Read the model definition and answer for the solid it produces. Units are mm, in the model's axes. Face numbers are marked on the shaded views. Round coordinates to 2 decimals unless told otherwise and drop trailing zeros. Loops run counter-clockwise (first coordinate to the right, second up) from the corner with the lowest first, then second, coordinate; pieces in that order, holes last. Notation, with made-up numbers: M -22,-33 L -9,-33 A23 ccw -9,1 Z; hole C 7,-14.75 d1. An arc over 180 degrees is marked long. Write each question's results on one line, items separated by ' | '.
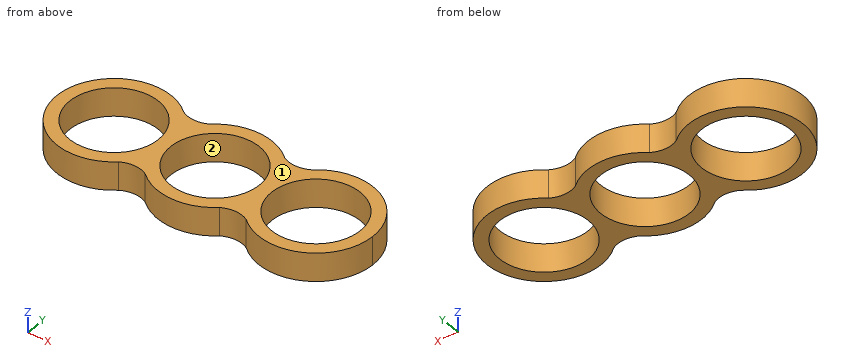
```python
from build123d import *

# Parameters (mm, degrees)
F0_R     = 11
F1_DEPTH = 7


with BuildPart() as f1:
    # F0 (on Top) → F1 (new body)
    with BuildSketch(Plane.XY):
        with BuildLine():
            ThreePointArc((-12.7, -6.29608), (-13.801325, -3.233274), (-14.175, 0))
            ThreePointArc((-14.175, 0), (-13.801325, 3.233274), (-12.7, 6.29608))
            ThreePointArc((-12.7, 6.29608), (-14.150621, 8.624506), (-16.022588, 10.6299))
            ThreePointArc((-16.022588, 10.6299), (-39.574997, 0.009606), (-16.037004, -10.6426))
            ThreePointArc((-16.037004, -10.6426), (-14.156468, -8.632127), (-12.7, -6.29608))
        make_face()
        with Locations((-25.4, 0)):
            Circle(F0_R, mode=Mode.SUBTRACT)
        with BuildLine():
            Line((11.225, 0), (11, 0))
            ThreePointArc((11, 0), (0, -11), (-11, 0))
            Line((-11, 0), (-11.225, 0))
            ThreePointArc((-11.225, 0), (-11.598675, -3.233274), (-12.7, -6.29608))
            ThreePointArc((-12.7, -6.29608), (-11.243532, -8.632127), (-9.362996, -10.6426))
            ThreePointArc((-9.362996, -10.6426), (0, -14.175), (9.362996, -10.6426))
            ThreePointArc((9.362996, -10.6426), (11.243532, -8.632127), (12.7, -6.29608))
            ThreePointArc((12.7, -6.29608), (11.598675, -3.233274), (11.225, 0))
        make_face()
        with BuildLine():
            ThreePointArc((-16.022588, 10.6299), (-14.150621, 8.624506), (-12.7, 6.29608))
            ThreePointArc((-12.7, 6.29608), (-11.243532, 8.632127), (-9.362996, 10.6426))
            ThreePointArc((-9.362996, 10.6426), (-12.691091, 9.744086), (-16.022588, 10.6299))
        make_face()
        with BuildLine():
            ThreePointArc((-12.7, -6.29608), (-11.598675, -3.233274), (-11.225, 0))
            Line((-11.225, 0), (-14.175, 0))
            ThreePointArc((-14.175, 0), (-13.801325, -3.233274), (-12.7, -6.29608))
        make_face()
        with BuildLine():
            Line((-14.175, 0), (-11.225, 0))
            ThreePointArc((-11.225, 0), (-11.598675, 3.233274), (-12.7, 6.29608))
            ThreePointArc((-12.7, 6.29608), (-13.801325, 3.233274), (-14.175, 0))
        make_face()
        with BuildLine():
            ThreePointArc((-11, 0), (0, 11), (11, 0))
            Line((11, 0), (11.225, 0))
            ThreePointArc((11.225, 0), (11.598675, 3.233274), (12.7, 6.29608))
            ThreePointArc((12.7, 6.29608), (11.243532, 8.632127), (9.362996, 10.6426))
            ThreePointArc((9.362996, 10.6426), (0, 14.175), (-9.362996, 10.6426))
            ThreePointArc((-9.362996, 10.6426), (-11.243532, 8.632127), (-12.7, 6.29608))
            ThreePointArc((-12.7, 6.29608), (-11.598675, 3.233274), (-11.225, 0))
            Line((-11.225, 0), (-11, 0))
        make_face()
        with BuildLine():
            ThreePointArc((-9.362996, -10.6426), (-11.243532, -8.632127), (-12.7, -6.29608))
            ThreePointArc((-12.7, -6.29608), (-14.156468, -8.632127), (-16.037004, -10.6426))
            ThreePointArc((-16.037004, -10.6426), (-12.7, -9.7536), (-9.362996, -10.6426))
        make_face()
        with BuildLine():
            ThreePointArc((16.037004, -10.6426), (14.156468, -8.632127), (12.7, -6.29608))
            ThreePointArc((12.7, -6.29608), (11.243532, -8.632127), (9.362996, -10.6426))
            ThreePointArc((9.362996, -10.6426), (12.7, -9.7536), (16.037004, -10.6426))
        make_face()
        with BuildLine():
            ThreePointArc((12.7, 6.29608), (13.801325, 3.233274), (14.175, 0))
            ThreePointArc((14.175, 0), (13.801325, -3.233274), (12.7, -6.29608))
            ThreePointArc((12.7, -6.29608), (14.156468, -8.632127), (16.037004, -10.6426))
            ThreePointArc((16.037004, -10.6426), (31.239955, -12.916096), (39.575, 0))
            ThreePointArc((39.575, 0), (31.239955, 12.916096), (16.037004, 10.6426))
            ThreePointArc((16.037004, 10.6426), (14.156468, 8.632127), (12.7, 6.29608))
        make_face()
        with BuildLine():
            ThreePointArc((36.4, 0), (25.4, -11), (14.4, 0))
            ThreePointArc((14.4, 0), (25.4, 11), (36.4, 0))
        make_face(mode=Mode.SUBTRACT)
        with BuildLine():
            ThreePointArc((12.7, 6.29608), (11.598675, 3.233274), (11.225, 0))
            Line((11.225, 0), (14.175, 0))
            ThreePointArc((14.175, 0), (13.801325, 3.233274), (12.7, 6.29608))
        make_face()
        with BuildLine():
            Line((14.175, 0), (11.225, 0))
            ThreePointArc((11.225, 0), (11.598675, -3.233274), (12.7, -6.29608))
            ThreePointArc((12.7, -6.29608), (13.801325, -3.233274), (14.175, 0))
        make_face()
        with BuildLine():
            ThreePointArc((9.362996, 10.6426), (11.243532, 8.632127), (12.7, 6.29608))
            ThreePointArc((12.7, 6.29608), (14.156468, 8.632127), (16.037004, 10.6426))
            ThreePointArc((16.037004, 10.6426), (12.7, 9.7536), (9.362996, 10.6426))
        make_face()
    extrude(amount=F1_DEPTH)


solid = f1.part
```
1. Find section C-C, the plane z = 2.75. Give the vertices of the cut face in (x, y) (3 decimals).
Completed:
outline: M -16.037,-10.643 A6.707 cw -9.363,-10.643 A14.175 ccw 9.363,-10.643 A6.707 cw 16.037,-10.643 A14.175 ccw 39.575,0 A14.175 ccw 16.037,10.643 A6.707 cw 9.363,10.643 A14.175 ccw -9.363,10.643 A6.66 cw -16.023,10.63 A14.175 ccw long Z; hole C -25.4,0 d22; hole C 0,0 d22; hole C 25.4,0 d22
2. Given P1, Ø4, axis at x = 19, z = 3.5, coming from the -Y side; P2, Ø2, axis at y = -2, z = 4.5, coming from the -X side, each flat-ended and moving along its own axis, determine where each tip first touches the part or whether it passes through.
Completed:
P1: stops at y = -13.47 | P2: stops at x = -39.54
3. Find section D-D, the plane x = 17. Give the vertices of the cut face in (y, z).
Completed:
outline: M -11.42,0 L -7.1,0 L -7.1,7 L -11.42,7 Z; M 7.1,0 L 11.42,0 L 11.42,7 L 7.1,7 Z
4. Determine the mould class of the marked faces 1 and 2 for opening direction X: released by +X, released by -X, zero draft, split by the parting line, or undercut.
Completed:
face 1: zero draft | face 2: undercut
5. Find the intervals of material crossed by L1, parallel to X at y = -9, z = 1; L2, parallel to X at y = -8.25, z = 6; L3, parallel to Y at x = 0, z = 3.75 (3 decimals), in increasing order.
Completed:
L1: x = -36.35 to -31.72, -19.08 to -6.32, 6.32 to 19.08, 31.72 to 36.35 | L2: x = -36.93 to -32.68, -18.12 to -7.28, 7.28 to 18.12, 32.68 to 36.93 | L3: y = -14.175 to -11, 11 to 14.175
6. Find section A-A, the plane x = -25.4. Give the vertices of the cut face in (y, z) (3 decimals), then the cut area to 4 significant figures.
Completed:
outline: M -14.175,0 L -11,0 L -11,7 L -14.175,7 Z; M 11,0 L 14.175,0 L 14.175,7 L 11,7 Z | area: 44.45 mm2
7. Find section B-B, the plane y = 5.75. Give the vertices of the cut face in (x, z).
Completed:
outline: M -38.36,0 L -34.78,0 L -34.78,7 L -38.36,7 Z; M -16.02,0 L -9.38,0 L -9.38,7 L -16.02,7 Z; M 9.38,0 L 16.02,0 L 16.02,7 L 9.38,7 Z; M 34.78,0 L 38.36,0 L 38.36,7 L 34.78,7 Z
